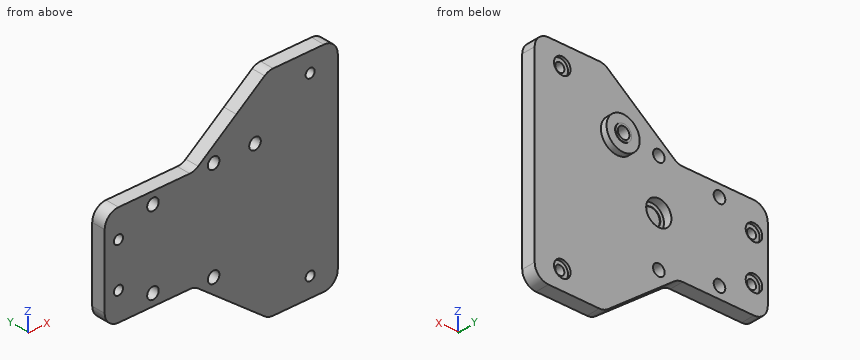
from build123d import *

# Parameters (mm, degrees)
SKETCH1_W           = 115
SKETCH1_H           = 60
SKETCH1_R           = 2.1
BOSS_EXTRUDE1_DEPTH = 5
SKETCH2_R           = 4.575
CUT_EXTRUDE1_DEPTH  = 3
SKETCH3_R           = 3.25
CUT_EXTRUDE2_DEPTH  = 0.2
SKETCH4_R           = 1.65
CUT_EXTRUDE3_DEPTH  = 6
CUT_EXTRUDE4_DEPTH  = 6
BOSS_EXTRUDE2_DEPTH = 5
SKETCH8_R           = 1.65
CUT_EXTRUDE5_DEPTH  = 6
FILLET1_R           = 5
SKETCH9_R           = 6
SKETCH9_R_2         = 2.1
BOSS_EXTRUDE3_DEPTH = 2.275
SKETCH10_R          = 2.9
SKETCH10_R_2        = 2.1
BOSS_EXTRUDE4_DEPTH = 0.2
SKETCH11_R          = 3
CUT_EXTRUDE6_DEPTH  = 1


with BuildPart() as part:
    # Sketch1 → Boss-Extrude1 (new body)
    with BuildSketch(Plane(origin=(0, 0, 0), x_dir=(1, 0, 0), z_dir=(0, 1, 0))):
        with Locations((-12.5, 0)):
            Rectangle(SKETCH1_W, SKETCH1_H)
        with Locations((-22, 14)):
            Circle(SKETCH1_R, mode=Mode.SUBTRACT)
        with Locations((0, 18)):
            Circle(SKETCH1_R, mode=Mode.SUBTRACT)
        with Locations((0, -18)):
            Circle(SKETCH1_R, mode=Mode.SUBTRACT)
        with Locations((-22, -14)):
            Circle(SKETCH1_R, mode=Mode.SUBTRACT)
        with Locations((15, -18)):
            Circle(SKETCH1_R, mode=Mode.SUBTRACT)
    extrude(amount=BOSS_EXTRUDE1_DEPTH)

    # Sketch2 → Cut-Extrude1 (cut)
    with BuildSketch(Plane(origin=(0, 5, 0), x_dir=(1, 0, 0), z_dir=(0, 1, 0))):
        Circle(SKETCH2_R)
    extrude(amount=-CUT_EXTRUDE1_DEPTH, mode=Mode.SUBTRACT)

    # Sketch3 → Cut-Extrude2 (cut)
    with BuildSketch(Plane(origin=(0, 2, 0), x_dir=(1, 0, 0), z_dir=(0, 1, 0))):
        Circle(SKETCH3_R)
    extrude(amount=-CUT_EXTRUDE2_DEPTH, mode=Mode.SUBTRACT)

    # Sketch4 → Cut-Extrude3 (cut, through all)
    with BuildSketch(Plane(origin=(0, 5, 0), x_dir=(1, 0, 0), z_dir=(0, 1, 0))):
        with Locations((-34.5, -8)):
            Circle(SKETCH4_R)
        with Locations((-34.5, 8)):
            Circle(SKETCH4_R)
    extrude(amount=-CUT_EXTRUDE3_DEPTH, mode=Mode.SUBTRACT)

    # Sketch6 → Cut-Extrude4 (cut, through all)
    with BuildSketch(Plane(origin=(0, 5, 0), x_dir=(1, 0, 0), z_dir=(0, 1, 0))):
        with BuildLine():
            Line((-22, 18.221576202), (-34.5, 18.221576202))
            ThreePointArc((-34.5, 18.221576202), (-38.035533906, 16.757110108), (-39.5, 13.221576202))
            Line((-39.5, 13.221576202), (-39.5, -13.221576202))
            ThreePointArc((-39.5, -13.221576202), (-38.035533906, -16.757110108), (-34.5, -18.221576202))
            Line((-34.5, -18.221576202), (-22, -18.221576202))
            Line((-22, -18.221576202), (-8.297519941, -18.221576202))
            Line((-8.297519941, -18.221576202), (-6.951019319, -18.221576202))
            Line((-6.951019319, -18.221576202), (19.301199277, -38.580439602))
            Line((19.301199277, -38.580439602), (-22, -30))
            Line((-22, -30), (-70, -30))
            Line((-70, -30), (-70, 30))
            Line((-70, 30), (-22, 30))
            Line((-22, 30), (19.301199277, 38.580439602))
            Line((19.301199277, 38.580439602), (-6.951019319, 18.221576202))
            Line((-6.951019319, 18.221576202), (-8.297519941, 18.221576202))
            Line((-8.297519941, 18.221576202), (-22, 18.221576202))
        make_face()
    extrude(amount=-CUT_EXTRUDE4_DEPTH, mode=Mode.SUBTRACT)

    # Sketch7 → Boss-Extrude2 (add)
    with BuildSketch(Plane(origin=(0, 5, 0), x_dir=(1, 0, 0), z_dir=(0, 1, 0))):
        Polygon((19.842211368, 39), (8.23694821, 30), (45, 30), (45, 39), align=None)
        Polygon((45, -30), (8.23694821, -30), (19.842211368, -39), (45, -39), align=None)
    extrude(amount=-BOSS_EXTRUDE2_DEPTH)

    # Sketch8 → Cut-Extrude5 (cut, through all)
    with BuildSketch(Plane(origin=(0, 5, 0), x_dir=(1, 0, 0), z_dir=(0, 1, 0))):
        with Locations((35, 32)):
            Circle(SKETCH8_R)
        with Locations((35, -32)):
            Circle(SKETCH8_R)
    extrude(amount=-CUT_EXTRUDE5_DEPTH, mode=Mode.SUBTRACT)

    # Fillet1
    fillet1_edges = [part.edges().sort_by_distance(p)[0] for p in [
        (45, 2.5, -39),
        (19.842211368, 2.5, -39),
        (19.842211368, 2.5, 39),
        (45, 2.5, 39),
        (-6.951019319, 2.5, 18.221576202),
        (-6.951019319, 2.5, -18.221576202),
    ]]
    fillet(fillet1_edges, radius=FILLET1_R)

    # Sketch9 → Boss-Extrude3 (add)
    with BuildSketch(Plane(origin=(0, 5, 0), x_dir=(1, 0, 0), z_dir=(0, 1, 0))):
        with Locations((15, -18)):
            Circle(SKETCH9_R)
        with Locations((15, -18)):
            Circle(SKETCH9_R_2, mode=Mode.SUBTRACT)
    extrude(amount=BOSS_EXTRUDE3_DEPTH)

    # Sketch10 → Boss-Extrude4 (add)
    with BuildSketch(Plane(origin=(0, 7.275, 0), x_dir=(1, 0, 0), z_dir=(0, 1, 0))):
        with Locations((15, -18)):
            Circle(SKETCH10_R)
        with Locations((15, -18)):
            Circle(SKETCH10_R_2, mode=Mode.SUBTRACT)
    extrude(amount=BOSS_EXTRUDE4_DEPTH)

    # Sketch11 → Cut-Extrude6 (cut)
    with BuildSketch(Plane(origin=(0, 5, 0), x_dir=(1, 0, 0), z_dir=(0, 1, 0))):
        with Locations((-34.5, 8)):
            Circle(SKETCH11_R)
        with Locations((-34.5, -8)):
            Circle(SKETCH11_R)
        with Locations((35, -32)):
            Circle(SKETCH11_R)
        with Locations((35, 32)):
            Circle(SKETCH11_R)
    extrude(amount=-CUT_EXTRUDE6_DEPTH, mode=Mode.SUBTRACT)


solid = part.part
Here's how the part is built. I have some questions about the finished solid (model axes, mm). Coordinates: 2 decimals unless noted, no trailing zeros. Write each loop counter-clockwise with the first axis right and the second up, starting at its lowest first coordinate (ties: lowest second). Pieces come first, ordered by that corner, then holes.
1) If we section it at C-C (x = 15.5): List the corners of the cut face in (y, z) for me (3 decimals).
Filled in:
outline: (0, -35.633) - (5, -35.633) - (5, 12.021) - (7.275, 12.021) - (7.275, 15.143) - (7.475, 15.143) - (7.475, 15.96) - (0, 15.96) - close; (0, 20.04) - (7.475, 20.04) - (7.475, 20.857) - (7.275, 20.857) - (7.275, 23.979) - (5, 23.979) - (5, 35.633) - (0, 35.633) - close
2) I'm going to push flat-ended pins straight in: pin 1 (6.5 mm diameter, centred on x = -34.5, z = -6.5, fed in from +Y); pin 2 (1.8 mm diameter, centred on x = -35.5, z = 6.5, fed in from +Y); pin 3 (3.5 mm diameter, centred on x = -22, z = 14, fed in from -Y). Where does each tip first touch, or does it pass through?
Filled in:
pin 1: stops at y = 5
pin 2: stops at y = 4
pin 3: passes through
3) If we section it at B-B (x = 35): List the corners of the cut face in (y, z) for me.
Filled in:
outline: (0, -39) - (5, -39) - (5, -35) - (4, -35) - (4, -33.65) - (0, -33.65) - close; (0, -30.35) - (4, -30.35) - (4, -29) - (5, -29) - (5, 29) - (4, 29) - (4, 30.35) - (0, 30.35) - close; (0, 33.65) - (4, 33.65) - (4, 35) - (5, 35) - (5, 39) - (0, 39) - close
4) If we section it at A-A (z = -8): List the corners of the cut face in (x, y) for me, plus the area to 3 significant figures.
Filled in:
outline: (-39.5, 0) - (-36.15, 0) - (-36.15, 4) - (-37.5, 4) - (-37.5, 5) - (-39.5, 5) - close; (-32.85, 0) - (45, 0) - (45, 5) - (-31.5, 5) - (-31.5, 4) - (-32.85, 4) - close
area: 403 mm2
5) If I drill on line 1 (Z direction, x = -34.5, y = 0.9); line 2 (Z direction, x = 35, y = 4.5); line 3 (Z direction, x = 0, y = 3.85) (3 decimals), over which ranges is the centre line in solid material (lowest first)?
Filled in:
line 1: z = -18.22 to -9.65, -6.35 to 6.35, 9.65 to 18.22
line 2: z = -39 to -35, -29 to 29, 35 to 39
line 3: z = -23.612 to -20.1, -15.9 to -4.575, 4.575 to 15.9, 20.1 to 23.612
6) If we section it at D-D (x = 0): List the corners of the cut face in (y, z) for me (3 decimals).
Filled in:
outline: (0, -23.612) - (5, -23.612) - (5, -20.1) - (0, -20.1) - close; (0, -15.9) - (5, -15.9) - (5, -4.575) - (2, -4.575) - (2, -3.25) - (1.8, -3.25) - (1.8, 3.25) - (2, 3.25) - (2, 4.575) - (5, 4.575) - (5, 15.9) - (0, 15.9) - close; (0, 20.1) - (5, 20.1) - (5, 23.612) - (0, 23.612) - close
